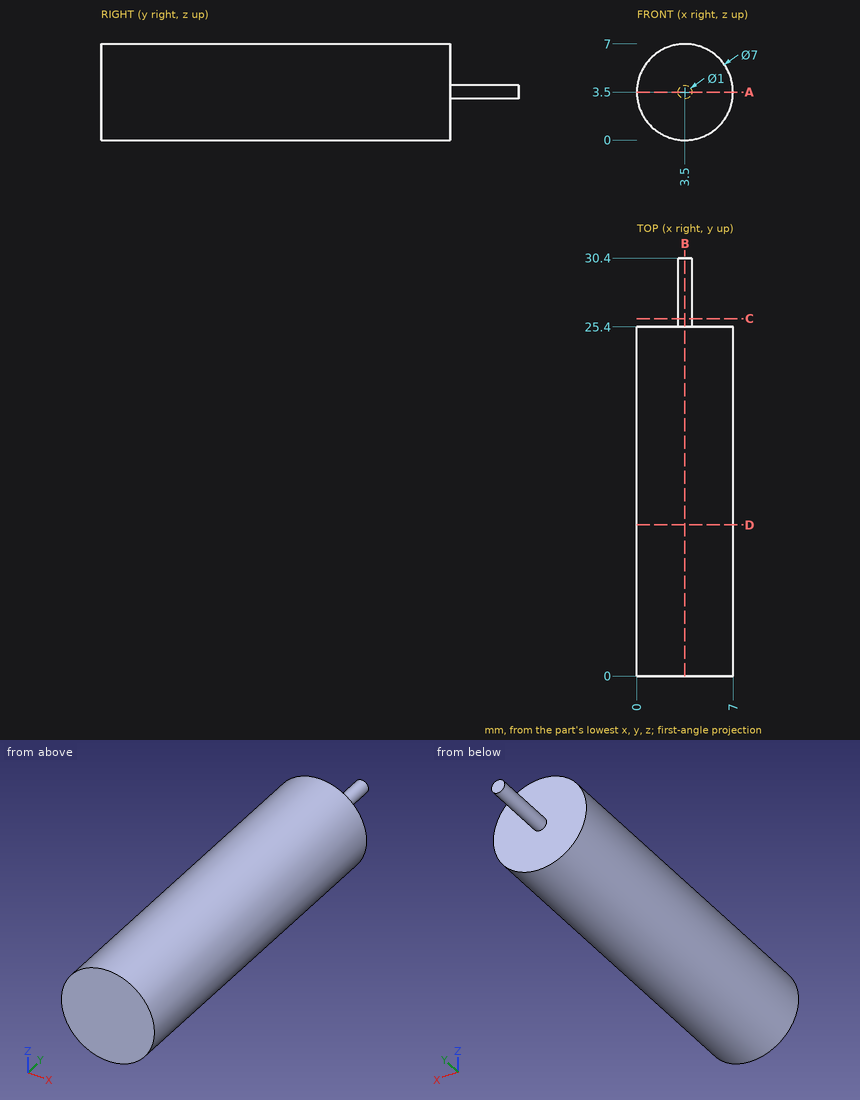
Can you work these out from the drawing? Everything is in mm from the part's minimum corner. Round coordinates to 2 decimals unless told otherwise and drop trailing zeros. Write each loop counter-clockwise with the first axis right and the second up, starting at its lowest first coordinate (ties: lowest second). Pieces come first, ordered by that corner, then holes.
1. Suppose I cut it at B-B (x = 3.5). List the corners of the cut face in (y, z) for me, and give its area (3 significant figures).
2. Will these pins go through, and if not, where does the flat tip stop? pin 1 Ø1.5 at (y, z) = (7, 6) entering from +X; pin 2 Ø2 at (x, z) = (6, 2) entering from +Y; pin 3 Ø2 at (x, z) = (3, 2.5) entering from -Y; pin 4 Ø1 at (y, z) = (23.5, 2) entering from -X.
3. Suppose I cut it at A-A (z = 3.5). List the corners of the cut face in (x, y) for me, and give its area (3 significant figures).
4. Suppose I cut it at C-C (y = 26). List the corners of the cut face in (x, z) for me.
5. Suppose I cut it at D-D (y = 11). List the corners of the cut face in (x, z) for me, and give its area (3 significant figures).
6. I need wall thicknesses on L1, parallel to Y at x = 2, z = 1; L2, parallel to X at y = 19.5, z = 2.5; L3, parallel to X at y = 16, z = 5. Which ranges of each line are inside material? Lowest first, please.
Answer sheet:
1. outline: (0, 0) - (25.4, 0) - (25.4, 3) - (30.4, 3) - (30.4, 4) - (25.4, 4) - (25.4, 7) - (0, 7) - close
1. area: 183 mm2
2. pin 1: stops at x = 6.53
2. pin 2: stops at y = 25.4
2. pin 3: stops at y = 0
2. pin 4: stops at x = 0.15
3. outline: (0, 0) - (7, 0) - (7, 25.4) - (4, 25.4) - (4, 30.4) - (3, 30.4) - (3, 25.4) - (0, 25.4) - close
3. area: 183 mm2
4. outline: circle Ø1 at (3.5, 3.5)
5. outline: circle Ø7 at (3.5, 3.5)
5. area: 38.5 mm2
6. L1: y = 0 to 25.4
6. L2: x = 0.15 to 6.85
6. L3: x = 0.34 to 6.66
